Drawing for the job (mm, zero at the part's lowest x, y, z). A direction names the side the tool comes from. Round coordinates to 2 decimals unless told otherwise and drop trailing zeros. Order: outer loops, then holes, each group sorted by start corner. A loop starts at its lowest first (then second) coordinate and runs counter-clockwise, first axis right, second up. Notation, with made-up numbers: (9.25, 81) -> (26.25, 81) arc R10 cw to (26.25, 95) -> close; hole circle Ø2 at (-16, 81.5). An arc over 180 degrees is marked (long way). Answer as CSV lines item,"result". Start each with the question number.
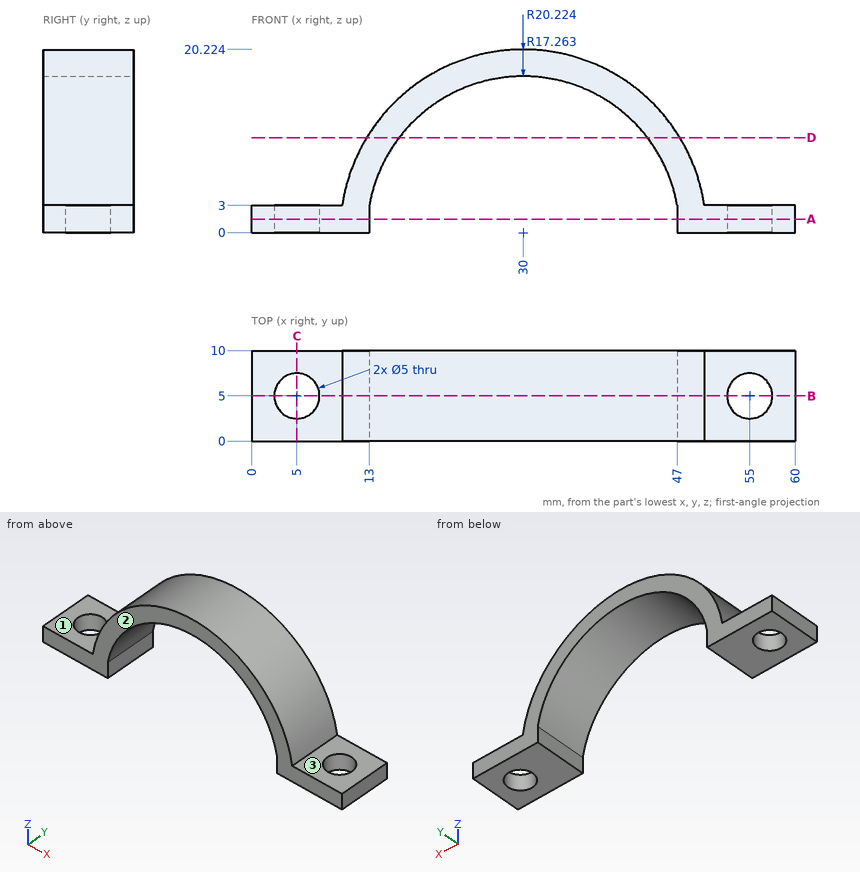
Q1. Which spindle directions (+Z, -Z, +X, -X, +Y, -Y) get a long thin tool onto all of the face, cutting with end or side? Do the marked faces 1, 2 and 3. Say none if no direction does.
Q2. Slice it at D-D, the plane z = 10.5. Write the cut outline in (x, y) (1 decimal).
Q3. Flat gauge pins, fed straight in: pin 1 Ø1 at (y, z) = (2, 14.5) entering from +X (1 decimal); pin 2 Ø5 at (x, y) = (57.5, 5) entering from +Z; pin 3 Ø6 at (x, y) = (20.5, 5) entering from +Z. Where does each tip first touch, or does it go through?
Q4. Slice it at A-A, the plane z = 1.5. Write the cut outline in (x, y), plus the area to 3 significant figures.
Q5. Slice it at B-B, the plane y = 5. Write the cut outline in (x, z) (1 decimal).
Q6. Slice it at C-C, the plane x = 5. Write the cut outline in (y, z), plus the area to 3 significant figures.
Q7. Probe L1, parallel to X at y = 5, z = 1.25; L2, parallel to Y at x = 5, z = 2.15; L3, parallel to X at y = 8.25, z = 11.25 (1 decimal). List the from-to ranges inside material, lowest first.
Solutions:
1,face 1,"+Z, -X, +Y, -Y"
1,face 2,"+Z, -Z, +X, -X, -Y"
1,face 3,"+Z, +X, +Y, -Y"
2,outline,"(12.7, 0) -> (16.3, 0) -> (16.3, 10) -> (12.7, 10) -> close; (43.7, 0) -> (47.3, 0) -> (47.3, 10) -> (43.7, 10) -> close"
3,pin 1,"stops at x = 44.6"
3,pin 2,"stops at z = 3"
3,pin 3,"stops at z = 19.15"
4,outline,"(0, 0) -> (13, 0) -> (13, 10) -> (0, 10) -> close; (47, 0) -> (60, 0) -> (60, 10) -> (47, 10) -> close; hole circle Ø5 at (5, 5); hole circle Ø5 at (55, 5)"
4,area,"221 mm2"
5,outline,"(0, 0) -> (2.5, 0) -> (2.5, 3) -> (0, 3) -> close; (7.5, 0) -> (13, 0) -> (13, 3) arc R17.3 cw to (47, 3) -> (47, 0) -> (52.5, 0) -> (52.5, 3) -> (50, 3) arc R20.2 ccw to (10, 3) -> (7.5, 3) -> close; (57.5, 0) -> (60, 0) -> (60, 3) -> (57.5, 3) -> close"
6,outline,"(0, 0) -> (2.5, 0) -> (2.5, 3) -> (0, 3) -> close; (7.5, 0) -> (10, 0) -> (10, 3) -> (7.5, 3) -> close"
6,area,"15.0 mm2"
7,L1,"x = 0 to 2.5, 7.5 to 13, 47 to 52.5, 57.5 to 60"
7,L2,"y = 0 to 2.5, 7.5 to 10"
7,L3,"x = 13.2 to 16.9, 43.1 to 46.8"
